Autodesk Inventor part; units mm, degrees
ref_plane "YZ Plane" through (0, 0, 0) normal (1, 0, 0) x (0, 1, 0)
ref_plane "XZ Plane" through (0, 0, 0) normal (0, 1, 0) x (-1, 0, 0)
ref_plane "XY Plane" through (0, 0, 0) normal (0, 0, 1) x (1, 0, 0)
sketch "Sketch_1" plane through (0, 0, 0) normal (0, 0, 1) x (1, 0, 0)
  line L0 (20, 0) -> (0, 0)
  line L1 (0, 0) -> (0, 3.5)
  line L2 (0, 3.5) -> (0.5, 4)
  line L3 (0.5, 4) -> (19.5, 4)
  line L4 (19.5, 4) -> (20, 3.5)
  line L5 (20, 3.5) -> (20, 0)
  line L6 (20, 0) -> (0, 0)
revolve "Revolution1" add sketch "Sketch_1" angle 360 about axis through (20, 0, 0) along (1, 0, 0)
sketch "Sketch2" plane through (0, 0, 0) normal (-1, 0, 0) x (0, 0, 1)
  point P0 (0, 0)
hole "Hole1" at (0, 0, 0) direction (1, 0, 0) diameter 3.242 depth 29.0641 tip angle 120 countersink diameter 4 countersink angle 90
sketch "_____16" plane through (0, 0, 0) normal (0, 0, 1) x (1, 0, 0)
  line L0 (20, 0) -> (-10, 0)
  line L1 (-10, 0) -> (-9.0641, 1.621)
  line L2 (-9.0641, 1.621) -> (19.621, 1.621)
  line L3 (19.621, 1.621) -> (20, 2)
  line L4 (20, 2) -> (20, 0)
  line L5 (20, 0) -> (-10, 0)
revolve "Revolution2" cut sketch "_____16" angle 360 about axis through (20, 0, 0) along (1, 0, 0)
thread "Thread1"
properties part number "SFHRW8-20-M4-N4_s" material "鋼、炭素鋼"
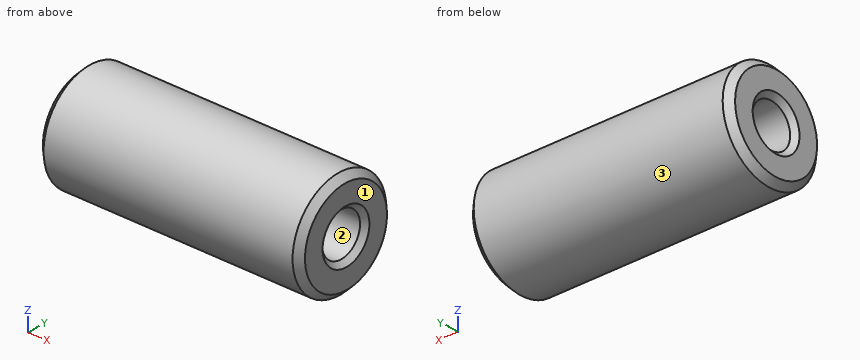
Read the model definition and answer for the solid it produces. Units are mm, in the model's axes. Face numbers are marked on the shaded views. Coordinates: 2 decimals unless noted, no trailing zeros. Order: outer loops, then holes, each group sorted by start corner. A loop starts at its lowest first (then second) coordinate and runs counter-clockwise, first axis right, second up. Notation, with made-up numbers: (43.25, 12) - (79.25, 12) arc R25 cw to (79.25, 49) - close; hole circle Ø4 at (-1.75, -31.5). An arc over 180 degrees is marked (long way). Use one line per item in the form item = value.
(1) For a pull along Z with two mould halves and no side action, classify the marked faces 1, 2 and 3 as pulls with the +Z half, pulls with the -Z half, needs draft (parallel to the pull), parting line crosses it, or undercut.
Computed values:
face_1 = needs draft
face_2 = undercut
face_3 = parting line crosses it
(2) Straight lines are drawn through the part: L1, parallel to Z at x = 15.75, y = 0; L2, parallel to Z at x = 9.75, y = -1; L3, parallel to Y at x = 12.5, z = -0.25. For each, find the intervals that lie inside material, in ascending order.
Computed values:
L1 = -4 to -1.62, 1.62 to 4
L2 = -3.87 to -1.28, 1.28 to 3.87
L3 = -3.99 to -1.6, 1.6 to 3.99
(3) Given pin 1 Ø2 at (x, z) = (14, -3) entering from -Y; pin 2 Ø2.5 at (y, z) = (0, 0) entering from +X (3 decimals), each flat-ended and moving along its own axis, determine where each tip first touches the part or whether it passes through.
Computed values:
pin_1 = -3.46
pin_2 = through
(4) Section B-B, the plane x = 6.75 is taken. Give the vertices of the cut face in (y, z).
Computed values:
outline = circle Ø8 at (0, 0); hole circle Ø3.24 at (0, 0)
(5) Section A-A, the plane z = 0 is taken. Give the vertices of the cut face in (x, y).
Computed values:
outline = (0, -3.5) - (0.5, -4) - (19.5, -4) - (20, -3.5) - (20, -2) - (19.62, -1.62) - (0.38, -1.62) - (0, -2) - close; (0, 2) - (0.38, 1.62) - (19.62, 1.62) - (20, 2) - (20, 3.5) - (19.5, 4) - (0.5, 4) - (0, 3.5) - close
